```python
from build123d import *

# Parameters (mm, degrees)
SKETCH1_R           = 6.477
BOSS_EXTRUDE1_DEPTH = 2.032
CUT_EXTRUDE1_DEPTH  = 0.64008
SKETCH3_W           = 1.19888
SKETCH3_H           = 8.98144
CUT_EXTRUDE2_DEPTH  = 1.09982
SKETCH4_W           = 7.19836
SKETCH4_H           = 7.00786
CUT_EXTRUDE3_DEPTH  = 0.8001
BOSS_EXTRUDE2_DEPTH = 1.27
SKETCH6_W           = 2.286
SKETCH6_H           = 1.99898
BOSS_EXTRUDE3_DEPTH = 2.54
SKETCH7_R           = 2.38125
BOSS_EXTRUDE4_DEPTH = 2.032


with BuildPart() as part:
    # Sketch1 → Boss-Extrude1 (new body)
    with BuildSketch(Plane(origin=(0, 0, 0), x_dir=(1, 0, 0), z_dir=(0, 1, 0))):
        with BuildLine():
            Line((-14.3002, 5.9944), (-14.3002, -24.3332))
            Line((-14.3002, -24.3332), (-9.271, -28.0416))
            Line((-9.271, -28.0416), (9.271, -28.0416))
            Line((9.271, -28.0416), (14.3002, -24.3332))
            Line((14.3002, -24.3332), (14.3002, 5.9944))
            ThreePointArc((14.3002, 5.9944), (0, 15.505758653), (-14.3002, 5.9944))
        make_face()
        with Locations(Location((0, 0, 0), (0, 0, 270))):
            Circle(SKETCH1_R, mode=Mode.SUBTRACT)
    extrude(amount=BOSS_EXTRUDE1_DEPTH)

    # Sketch2 → Cut-Extrude1 (cut)
    with BuildSketch(Plane(origin=(0, 2.032, 0), x_dir=(1, 0, 0), z_dir=(0, 1, 0))):
        Polygon((0, -28.0416), (-7.71906, -28.0416), (-7.71906, -16.06042), (7.71906, -16.06042), (7.71906, -28.0416), align=None)
    extrude(amount=-CUT_EXTRUDE1_DEPTH, mode=Mode.SUBTRACT)

    # Sketch3 → Cut-Extrude2 (cut)
    with BuildSketch(Plane(origin=(0, 1.39192, 0), x_dir=(1, 0, 0), z_dir=(0, 1, 0))):
        with Locations((-5.06984, -23.55088)):
            Rectangle(SKETCH3_W, SKETCH3_H)
        with Locations((2.52984, -23.55088)):
            Rectangle(SKETCH3_W, SKETCH3_H)
    extrude(amount=-CUT_EXTRUDE2_DEPTH, mode=Mode.SUBTRACT)

    # Sketch4 → Cut-Extrude3 (cut)
    with BuildSketch(Plane(origin=(0, 2.032, 0), x_dir=(1, 0, 0), z_dir=(0, 1, 0))):
        with Locations((-3.299968, -11.116564)):
            Rectangle(SKETCH4_W, SKETCH4_H)
    extrude(amount=-CUT_EXTRUDE3_DEPTH, mode=Mode.SUBTRACT)

    # Sketch5 → Boss-Extrude2 (add)
    with BuildSketch(Plane(origin=(0, 2.032, 0), x_dir=(1, 0, 0), z_dir=(0, 1, 0))):
        with BuildLine():
            Line((12.40282, -22.33422), (13.171678, -22.33422))
            Line((13.171678, -22.33422), (13.40104, -22.152864))
            Line((13.40104, -22.152864), (13.40104, 4.882896))
            ThreePointArc((13.40104, 4.882896), (13.360125716, 5.283490726), (13.23975, 5.667756))
            ThreePointArc((13.23975, 5.667756), (10.160746855, 10.20631074), (5.608066, 13.264388))
            ThreePointArc((5.608066, 13.264388), (5.250053957, 13.366581837), (4.87934, 13.40104))
            Line((4.87934, 13.40104), (4.50342, 13.40104))
            Line((4.50342, 13.40104), (4.50342, 12.40282))
            Line((4.50342, 12.40282), (4.87934, 12.40282))
            ThreePointArc((4.87934, 12.40282), (5.080028543, 12.382451063), (5.272532, 12.322175))
            ThreePointArc((5.272532, 12.322175), (9.477779109, 9.479294357), (12.322175, 5.275072))
            ThreePointArc((12.322175, 5.275072), (12.382451063, 5.082568543), (12.40282, 4.88188))
            Line((12.40282, 4.88188), (12.40282, -22.33422))
        make_face()
        with BuildLine():
            Line((-4.850750436, 13.40104), (-4.474830436, 13.40104))
            Line((-4.474830436, 13.40104), (-4.474830436, 12.40282))
            Line((-4.474830436, 12.40282), (-4.850750436, 12.40282))
            ThreePointArc((-4.850750436, 12.40282), (-5.051438979, 12.382451063), (-5.243942436, 12.322175))
            ThreePointArc((-5.243942436, 12.322175), (-9.449189546, 9.479294357), (-12.293585436, 5.275072))
            ThreePointArc((-12.293585436, 5.275072), (-12.353861499, 5.082568543), (-12.374230436, 4.88188))
            Line((-12.374230436, 4.88188), (-12.374230436, -22.33422))
            Line((-12.374230436, -22.33422), (-13.143088436, -22.33422))
            Line((-13.143088436, -22.33422), (-13.372450436, -22.152864))
            Line((-13.372450436, -22.152864), (-13.372450436, 4.882896))
            ThreePointArc((-13.372450436, 4.882896), (-13.331536152, 5.283490726), (-13.211160436, 5.667756))
            ThreePointArc((-13.211160436, 5.667756), (-10.132157291, 10.20631074), (-5.579476436, 13.264388))
            ThreePointArc((-5.579476436, 13.264388), (-5.221464393, 13.366581837), (-4.850750436, 13.40104))
        make_face()
    extrude(amount=BOSS_EXTRUDE2_DEPTH)

    # Sketch6 → Boss-Extrude3 (add)
    with BuildSketch(Plane(origin=(0, 1.39192, 0), x_dir=(1, 0, 0), z_dir=(0, 1, 0))):
        with Locations((6.57606, -27.04211)):
            Rectangle(SKETCH6_W, SKETCH6_H)
    extrude(amount=BOSS_EXTRUDE3_DEPTH)

    # Sketch7 → Boss-Extrude4 (add)
    with BuildSketch(Plane.XZ):
        with BuildLine():
            ThreePointArc((-12.144798566, -9.640146223), (-11.377973728, -11.033206497), (-11.1125, -12.601058837))
            Line((-11.1125, -12.601058837), (-11.1125, -19.05))
            ThreePointArc((-11.1125, -19.05), (-9.717596045, -22.417596045), (-6.35, -23.8125))
            Line((-6.35, -23.8125), (-5.983425441, -23.8125))
            ThreePointArc((-5.983425441, -23.8125), (-4.22646321, -23.476566386), (-2.717363519, -22.516157205))
            ThreePointArc((-2.717363519, -22.516157205), (0, -21.4376), (2.717363519, -22.516157205))
            ThreePointArc((2.717363519, -22.516157205), (4.22646321, -23.476566386), (5.983425441, -23.8125))
            Line((5.983425441, -23.8125), (6.35, -23.8125))
            ThreePointArc((6.35, -23.8125), (9.717596045, -22.417596045), (11.1125, -19.05))
            Line((11.1125, -19.05), (11.1125, -12.601058837))
            ThreePointArc((11.1125, -12.601058837), (11.377973728, -11.033206497), (12.144798566, -9.640146223))
            ThreePointArc((12.144798566, -9.640146223), (0, -15.505758653), (-12.144798566, -9.640146223))
        make_face()
        with Locations(Location((-6.35, -19.05, 0), (0, 0, 270))):
            Circle(SKETCH7_R, mode=Mode.SUBTRACT)
        with Locations(Location((6.35, -19.05, 0), (0, 0, 270))):
            Circle(SKETCH7_R, mode=Mode.SUBTRACT)
    extrude(amount=-BOSS_EXTRUDE4_DEPTH)


solid = part.part
```
Build history of the part. All positions in model axes, mm. A direction names the side the tool comes from. Give positions to 0.01 mm unless a question says otherwise; leave off trailing zeros. Loops run counter-clockwise (first coordinate to the right, second up) from the corner with the lowest first, then second, coordinate; pieces in that order, holes last.
Item 1: Slice it at A-A, the plane z = 0. List the corners of the cut face in (x, y).
Answers follow:
outline: (-14.3, 0) - (-6.48, 0) - (-6.48, 2.03) - (-12.37, 2.03) - (-12.37, 3.3) - (-13.37, 3.3) - (-13.37, 2.03) - (-14.3, 2.03) - close; (6.48, 0) - (14.3, 0) - (14.3, 2.03) - (13.4, 2.03) - (13.4, 3.3) - (12.4, 3.3) - (12.4, 2.03) - (6.48, 2.03) - close
Item 2: Slice it at C-C, the plane x = 7. List the corners of the cut face in (y, z).
Answers follow:
outline: (0, -23.77) - (2.03, -23.77) - (2.03, -21.34) - (0, -21.34) - close; (0, -16.76) - (2.03, -16.76) - (2.03, -12.59) - (3.3, -12.59) - (3.3, -11.43) - (2.03, -11.43) - (2.03, 16.06) - (1.39, 16.06) - (1.39, 26.04) - (3.93, 26.04) - (3.93, 28.04) - (0, 28.04) - close
Item 3: Drill centre lines: line 1 (X direction, y = 0.75, z = -19.05); line 2 (X direction, y = 0.55, z = 21.5); line 3 (X direction, y = 3, z = 19.5). Where is each one in solid material? Low to high.
Answers follow:
line 1: x = -11.11 to -8.73, -3.97 to 3.97, 8.73 to 11.11
line 2: x = -14.3 to -5.67, -4.47 to 1.93, 3.13 to 14.3
line 3: x = -13.37 to -12.37, 12.4 to 13.4
Item 4: Slice it at B-B, the plane z = 14. List the corners of the cut face in (x, y).
Answers follow:
outline: (-14.3, 0) - (14.3, 0) - (14.3, 2.03) - (13.4, 2.03) - (13.4, 3.3) - (12.4, 3.3) - (12.4, 2.03) - (0.3, 2.03) - (0.3, 1.23) - (-6.9, 1.23) - (-6.9, 2.03) - (-12.37, 2.03) - (-12.37, 3.3) - (-13.37, 3.3) - (-13.37, 2.03) - (-14.3, 2.03) - close
Item 5: Pull direction Z, two halves, no side cores. Call faces 1 (the face through (11.371, 1.002, -11.054)), 2 (the face through (-3, 1.232, 11)), 3 (the face through (9.427, 2.658, -9.53)), 4 (the face through (4.503, 3, -13)): released by +Z, released by -Z, zero draft, split by the parting line, or undercut.
Answers follow:
face 1: released by -Z
face 2: undercut
face 3: undercut
face 4: zero draft
Item 6: Flat gauge pins, fed straight in: pin 1 (2 mm diameter, centred on y = 2.5, z = 27, fed in from -X); pin 2 (0.7 mm diameter, centred on x = 6, y = 2.5, fed in from -Z); pin 3 (2 mm diameter, centred on y = 2, z = -11.5, fed in from -X). Where does each tip first touch, or does it go through?
Answers follow:
pin 1: stops at x = -11.88
pin 2: stops at z = -13.25
pin 3: stops at x = -11.6
Item 7: Which spindle directions (+Z, -Z, +X, -X, +Y, -Y) get a long thin tool onto all of the face, cutting with end or side? Do faces 5 (the face through (-4.475, 3, -13)), 6 (the face through (-5, 0.292, 23)), 7 (the face through (7.719, 3, 27)), 8 (the face through (-10.19, 2.66, -10.15)). Say none if no direction does.
Answers follow:
face 5: +Z, -Z, +Y
face 6: +Z, +Y
face 7: +Z, +X, +Y
face 8: -Z, -X, +Y
Item 8: Slice it at D-D, the plane z = -17.5. List the corners of the cut face in (x, y).
Answers follow:
outline: (-11.11, 0) - (-8.16, 0) - (-8.16, 2.03) - (-11.11, 2.03) - close; (-4.54, 0) - (4.54, 0) - (4.54, 2.03) - (-4.54, 2.03) - close; (8.16, 0) - (11.11, 0) - (11.11, 2.03) - (8.16, 2.03) - close
